For this review, take the finished solid that the model builds, in its own axes (mm). A direction names the side the tool comes from. Coordinates: 2 decimals unless noted, no trailing zeros. Loops run counter-clockwise (first coordinate to the right, second up) from the corner with the lowest first, then second, coordinate; pieces in that order, holes last. Notation, with made-up numbers: (30.5, -23) - (88.5, -23) arc R16 cw to (88.5, -19) - close; hole circle Ø7 at (20, -10). An arc over 180 degrees is marked (long way). One line per item, written item: value. Start each with the question number.
1. Take a section at B-B, the plane z = 0. State the section outline as (x, y) points, and give its area (3 significant figures).
2. For faces 4 (the face through (-10.7, 2.54, 0.11)), 5 (the face through (-7, 5, 7)), list the 3-axis set-ups (+Z, -Z, +X, -X, +Y, -Y) from which the entire face can be reached by the end or side of a thin tool; tool diameter is ignored.
3. Take a section at A-A, the plane x = 0. State the section outline as (y, z) points.
4. Take a section at C-C, the plane y = 0.7. State the section outline as (x, z) points.
5. The part is to be moulded in two halves that separate along Z. For faces 1 (the face through (5.121, 2.465, 16.263)), 2 (the face through (-7, 0, 7)), 3 (the face through (-10.6, 2.5, -1.4)), say which applies: released by +Z, released by -Z, zero draft, split by the parting line, or undercut.
6. To check wall thickness, follow line 1 (X direction, y = 3.5, z = 0); line 2 (Z direction, x = -8, y = 3.7); line 3 (Z direction, x = -1.5, y = 2.7). State the ranges of each line that lie inside material, in increasing order. Write a range as from..to.
7. Insertion check: pin 1 (8 mm diameter, centred on x = 5.5, z = 4.5, fed in from -Y); pin 2 (3 mm diameter, centred on x = 10, y = 1, fed in from +Z). Each pin has a flat end and moves straight along its axis. Give the tip position at first contact, or say it passes through.
8. Take a section at D-D, the plane z = 14.5. State the section outline as (x, y) points, and give its area (3 significant figures).
```python
from build123d import *

# Parameters (mm, degrees)
SKETCH_1_R          = 17.05
EXTRUDE_1_DEPTH     = 5
SKETCH_2_R          = 9.15
CUT_EXTRUDE_1_DEPTH = 5
CUT_EXTRUDE_2_DEPTH = 25.625291876


with BuildPart() as part:
    # 草圖1 → 填料-伸長1 (new body)
    with BuildSketch(Plane(origin=(0, 0, 0), x_dir=(1, 0, 0), z_dir=(0, 1, 0))):
        with Locations(Location((0, 0, 0), (0, 0, 270))):
            Circle(SKETCH_1_R)
    extrude(amount=EXTRUDE_1_DEPTH)

    # 草圖2 → 除料-伸長1 (cut)
    with BuildSketch(Plane(origin=(0, 5, 0), x_dir=(1, 0, 0), z_dir=(0, 1, 0))):
        with Locations(Location((0, 0, 0), (0, 0, 270))):
            Circle(SKETCH_2_R)
    extrude(amount=-CUT_EXTRUDE_1_DEPTH, mode=Mode.SUBTRACT)

    # 草圖3 → 除料-伸長2 (cut, through all)
    with BuildSketch(Plane(origin=(0, 5, 0), x_dir=(1, 0, 0), z_dir=(0, 1, 0))):
        Polygon((-10.647976509, 0.685197974), (-10.548439784, 2.231998685), (-8.899610355, 2.125896405), (-9.095873569, -0.993772622), (-10.74706795, -0.889893424), align=None)
    extrude(amount=-CUT_EXTRUDE_2_DEPTH, mode=Mode.SUBTRACT)


solid = part.part
```
Solutions:
1. outline: (-17.05, 0) - (-10.69, 0) - (-10.69, 5) - (-17.05, 5) - close; (9.15, 0) - (17.05, 0) - (17.05, 5) - (9.15, 5) - close
1. area: 71.3 mm2
2. face 4: +Y, -Y
2. face 5: +Z, -Z, +X, -X, +Y
3. outline: (0, -17.05) - (5, -17.05) - (5, -9.15) - (0, -9.15) - close; (0, 9.15) - (5, 9.15) - (5, 17.05) - (0, 17.05) - close
4. outline: circle Ø34.1 at (0, 0); hole (-10.75, 0.89) - (-10.65, -0.69) - (-10.55, -2.23) - (-8.9, -2.13) arc R9.15 ccw (long way) to (-9.1, 0.99) - close
5. face 1: split by the parting line
5. face 2: zero draft
5. face 3: undercut
6. line 1: -17.05..-10.69, 9.15..17.05
6. line 2: -15.06..-4.44, 4.44..15.06
6. line 3: -16.98..-9.03, 9.03..16.98
7. pin 1: y = 0
7. pin 2: z = 14.78
8. outline: (-8.97, 0) - (8.97, 0) - (8.97, 5) - (-8.97, 5) - close
8. area: 89.7 mm2
